```python
from build123d import *

# Parameters (mm, degrees)
SKETCH1_R           = 3.175
BOSS_EXTRUDE1_DEPTH = 19.05
SKETCH3_R           = 9.525
BOSS_EXTRUDE2_DEPTH = 12.7
SKETCH4_R           = 3.175
CUT_EXTRUDE1_DEPTH  = 67.599361859


with BuildPart() as part:
    # Sketch1 → Boss-Extrude1 (new body)
    with BuildSketch(Plane(origin=(0, 0, 0), x_dir=(1, 0, 0), z_dir=(0, 1, 0))):
        with BuildLine():
            Line((-38.1, 31.75), (38.1, 31.75))
            ThreePointArc((38.1, 31.75), (42.590128061, 29.890128061), (44.45, 25.4))
            Line((44.45, 25.4), (44.45, -25.4))
            ThreePointArc((44.45, -25.4), (42.590128061, -29.890128061), (38.1, -31.75))
            Line((38.1, -31.75), (-38.1, -31.75))
            ThreePointArc((-38.1, -31.75), (-42.590128061, -29.890128061), (-44.45, -25.4))
            Line((-44.45, -25.4), (-44.45, 25.4))
            ThreePointArc((-44.45, 25.4), (-42.590128061, 29.890128061), (-38.1, 31.75))
        make_face()
        with Locations(Location((-38.1, 25.4, 0), (0, 0, 90))):
            Circle(SKETCH1_R, mode=Mode.SUBTRACT)
        with Locations(Location((-38.1, -25.4, 0), (0, 0, 90))):
            Circle(SKETCH1_R, mode=Mode.SUBTRACT)
        with Locations(Location((38.1, -25.4, 0), (0, 0, 90))):
            Circle(SKETCH1_R, mode=Mode.SUBTRACT)
        with Locations(Location((38.1, 25.4, 0), (0, 0, 90))):
            Circle(SKETCH1_R, mode=Mode.SUBTRACT)
    extrude(amount=BOSS_EXTRUDE1_DEPTH)

    # Sketch3 → Boss-Extrude2 (add, symmetric)
    with BuildSketch(Plane(origin=(0, 0, 0), x_dir=(0, 1, 0), z_dir=(-0.500000000000001, 0, -0.866025403784438))):
        with BuildLine():
            Line((25.4, 19.048282487), (19.05, 19.048282487))
            Line((19.05, 19.048282487), (19.05, 17.120567884))
            Line((19.05, 17.120567884), (19.05, -19.048282487))
            Line((19.05, -19.048282487), (25.4, -19.048282487))
            Line((25.4, -19.048282487), (25.4, -12.698282487))
            Line((25.4, -12.698282487), (31.75, -12.698282487))
            Line((31.75, -12.698282487), (31.75, -19.048282487))
            Line((31.75, -19.048282487), (38.1, -19.048282487))
            ThreePointArc((38.1, -19.048282487), (56.894198738, 0), (38.1, 19.048282487))
            Line((38.1, 19.048282487), (31.75, 19.048282487))
            Line((31.75, 19.048282487), (31.75, 12.698282487))
            Line((31.75, 12.698282487), (25.4, 12.698282487))
            Line((25.4, 12.698282487), (25.4, 19.048282487))
        make_face()
        with Locations(Location((37.844198738, 0, 0), (0, 0, 270))):
            Circle(SKETCH3_R, mode=Mode.SUBTRACT)
    extrude(amount=BOSS_EXTRUDE2_DEPTH, both=True)

    # Sketch4 → Cut-Extrude1 (cut, through all)
    with BuildSketch(Plane(origin=(0, 38.1, 0), x_dir=(1, 0, 0), z_dir=(0, 1, 0))):
        with Locations(Location((0, 0, 0), (0, 0, 90))):
            Circle(SKETCH4_R)
    extrude(amount=CUT_EXTRUDE1_DEPTH, mode=Mode.SUBTRACT)


solid = part.part
```
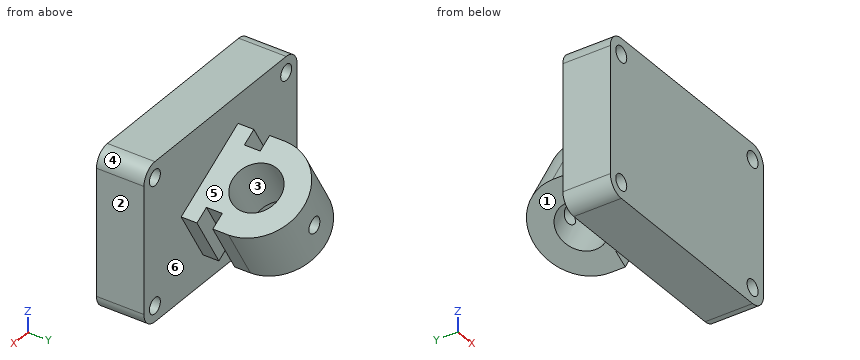
Could you check a few things on this model? Use its own coordinates, in mm. Face numbers are marked on the shaded views. A direction names the side the tool comes from. Round coordinates to 2 decimals unless told otherwise and drop trailing zeros. Write each loop counter-clockwise with the first axis right and the second up, starting at its lowest first coordinate (ties: lowest second). Pieces come first, ordered by that corner, then holes.
(1) Suppose I cut it at B-B on y = 17. Write out the boundary of the cut face in (x, z) (3 decimals).
Findings below:
outline: (-44.45, -25.4) arc R6.35 ccw to (-38.1, -31.75) - (38.1, -31.75) arc R6.35 ccw to (44.45, -25.4) - (44.45, 25.4) arc R6.35 ccw to (38.1, 31.75) - (-38.1, 31.75) arc R6.35 ccw to (-44.45, 25.4) - close; hole circle Ø6.35 at (-38.1, -25.4); hole circle Ø6.35 at (-38.1, 25.4); hole circle Ø6.35 at (38.1, -25.4); hole circle Ø6.35 at (38.1, 25.4)
(2) Which directions (+Z, -Z, +X, -X, +Y, -Y) give clear straight access to the entire face, cutting with the end or side of a thin tool? Please do the marked faces 4, 5 and 6.
Findings below:
face 4: +Z, +X, +Y, -Y
face 5: +Z, +X, +Y
face 6: +Y
(3) Thinking about a two-plate mould opening in Z: for the marked faces 1, 2 and 3, which applies, +Z half, -Z half, draft (parallel to the pull), parting line (faces both ways), or undercut?
Findings below:
face 1: -Z half
face 2: draft
face 3: undercut
(4) If I drill on probe 1 along Z at (x, y) = (38.1, 12.25) (3 decimals); probe 2 along X at (y, z) = (10, 25.4) (3 decimals), over which ranges is the centre line in solid material (lowest first)?
Findings below:
probe 1: z = -31.75 to -28.575, -22.225 to 22.225, 28.575 to 31.75
probe 2: x = -44.45 to -41.275, -34.925 to 34.925, 41.275 to 44.45
(5) For pin 1 (5 mm diameter, centred on x = 17, y = 32.5, fed in from -Z); pin 2 (5.5 mm diameter, centred on x = 10.5, z = -3.5, fed in from +Y); pin 3 (5 mm diameter, centred on x = -34, z = 16.5, fed in from +Y), each with a flat end and sliding along its axis, tell me the tip position at first contact or that it passes through.
Findings below:
pin 1: stops at z = -12.98
pin 2: stops at y = 55.09
pin 3: stops at y = 19.05
(6) Suppose I cut it at C-C on x = 0. State how many separate pieces and enclosed holes the cut face has, and give its area (3 significant figures).
Findings below:
separate pieces: 3
enclosed holes: 0
area: 1,750 mm2
(7) Suppose I cut it at A-A on x = -37. Write out the boundary of the cut face in (y, z).
Findings below:
outline: (0, -31.75) - (19.05, -31.75) - (19.05, -28.38) - (0, -28.38) - close; (0, -22.42) - (19.05, -22.42) - (19.05, 22.42) - (0, 22.42) - close; (0, 28.38) - (19.05, 28.38) - (19.05, 31.75) - (0, 31.75) - close
